CAD build for the part. Positions are in the model's coordinates, mm. Give positions to 0.01 mm unless a question says otherwise; leave off trailing zeros. Write each loop counter-clockwise with the first axis right and the second up, starting at its lowest first coordinate (ties: lowest second). Pieces come first, ordered by that corner, then holes. Notation, with made-up numbers: (-6, 19.25) -> (43, 19.25) arc R30 cw to (43, 49.25) -> close; hole circle Ø5 at (66.25, 59). An arc over 180 degrees is marked (long way). Answer as a JSON object with one key per item and string values.
```python
from build123d import *

# Parameters (mm, degrees)
SKETCH1_R           = 21.5
SKETCH1_R_2         = 7
BOSS_EXTRUDE1_DEPTH = 3.175
SKETCH2_R           = 1.625
CUT_EXTRUDE1_DEPTH  = 84.415110292


with BuildPart() as part:
    # Sketch1 → Boss-Extrude1 (new body)
    with BuildSketch(Plane(origin=(0, 0, 0), x_dir=(0, 0, -1), z_dir=(1, 0, 0))):
        with BuildLine():
            Line((-5.724395537, 29.448791074), (57.710241785, 41.77951643))
            ThreePointArc((57.710241785, 41.77951643), (70.733126292, 35.366563146), (68.049758215, 21.10048357))
            Line((68.049758215, 21.10048357), (20.124395537, -22.248791074))
            ThreePointArc((20.124395537, -22.248791074), (-26.83281573, -13.416407865), (-5.724395537, 29.448791074))
        make_face()
        Circle(SKETCH1_R, mode=Mode.SUBTRACT)
        with Locations((60, 30)):
            Circle(SKETCH1_R_2, mode=Mode.SUBTRACT)
    extrude(amount=BOSS_EXTRUDE1_DEPTH)

    # Sketch2 → Cut-Extrude1 (cut, through all)
    with BuildSketch(Plane(origin=(3.175, 0, 0), x_dir=(0, 0, -1), z_dir=(1, 0, 0))):
        with Locations((-20.175789947, 16)):
            Circle(SKETCH2_R)
        with Locations((16.003976299, 20.255101188)):
            Circle(SKETCH2_R)
        with Locations((20.259077487, -15.924665058)):
            Circle(SKETCH2_R)
        with Locations((-15.920688759, -20.179766246)):
            Circle(SKETCH2_R)
        with Locations((38.058110346, 0.174851372)):
            Circle(SKETCH2_R)
        with Locations((55.857143206, 16.274367802)):
            Circle(SKETCH2_R)
        with Locations(Location((22.974747305, 30.341577454, 0), (0, 0, 180))):
            Circle(SKETCH2_R)
        with Locations((34.754263735, 32.631335669)):
            Circle(SKETCH2_R)
    extrude(amount=-CUT_EXTRUDE1_DEPTH, mode=Mode.SUBTRACT)


solid = part.part
```
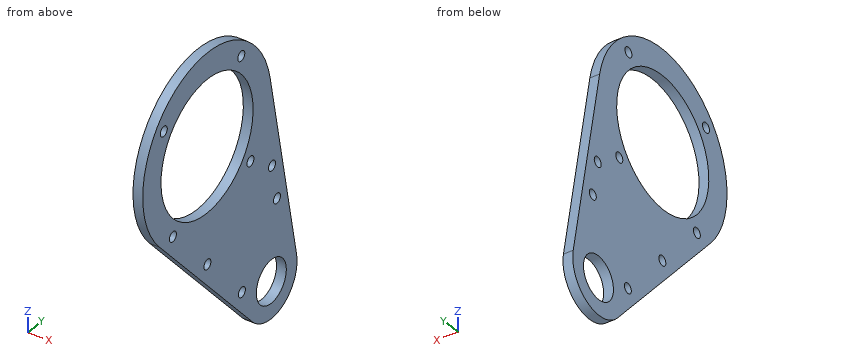
1) Slice it at A-A (y = -11). List the corners of the cut face in (x, z) (3 decimals).
Model answer:
{"outline": "(0, -32.561) -> (3.175, -32.561) -> (3.175, -18.473) -> (0, -18.473) -> close; (0, 18.473) -> (3.175, 18.473) -> (3.175, 27.911) -> (0, 27.911) -> close"}
2) Slice it at B-B (z = 4.5). List the corners of the cut face in (x, y) (3 decimals), then the cut area to 3 significant figures.
Model answer:
{"outline": "(0, -29.661) -> (3.175, -29.661) -> (3.175, -21.024) -> (0, -21.024) -> close; (0, 21.024) -> (3.175, 21.024) -> (3.175, 29.687) -> (0, 29.687) -> close", "area": "54.9 mm2"}
3) Wall check: probe 1 along Y at (x, z) = (2.65, 15); probe 2 along Y at (x, z) = (0.25, 14.5); probe 3 along Z at (x, y) = (1.6, -8). Give the ranges that are in metal, low to high.
Model answer:
{"probe 1": "y = -25.98 to -21.52, -18.84 to -15.4, 15.4 to 25.98", "probe 2": "y = -26.26 to -20.97, -19.39 to -15.87, 15.87 to 26.26", "probe 3": "z = -35.88 to -19.96, 19.96 to 28.91"}
4) Slice it at D-D (y = -26). List the corners of the cut face in (x, z) (3 decimals).
Model answer:
{"outline": "(0, -14.967) -> (3.175, -14.967) -> (3.175, 14.967) -> (0, 14.967) -> close"}
5) Slice it at C-C (x = 1.3). State how many separate pieces and enclosed holes the cut face has, then the cut area to 3 significant figures.
Model answer:
{"separate pieces": "1", "enclosed holes": "10", "area": "2,890 mm2"}
6) Pin check, flat tips, straight feed: pin 1 (3.5 mm diameter, centred on y = 32.63, z = -34.75, fed in from -X); pin 2 (1.5 mm diameter, centred on x = 1.5, z = -37, fed in from +Y). Stop position of each tip, or through.
Model answer:
{"pin 1": "stops at x = 0", "pin 2": "stops at y = 37.9"}
